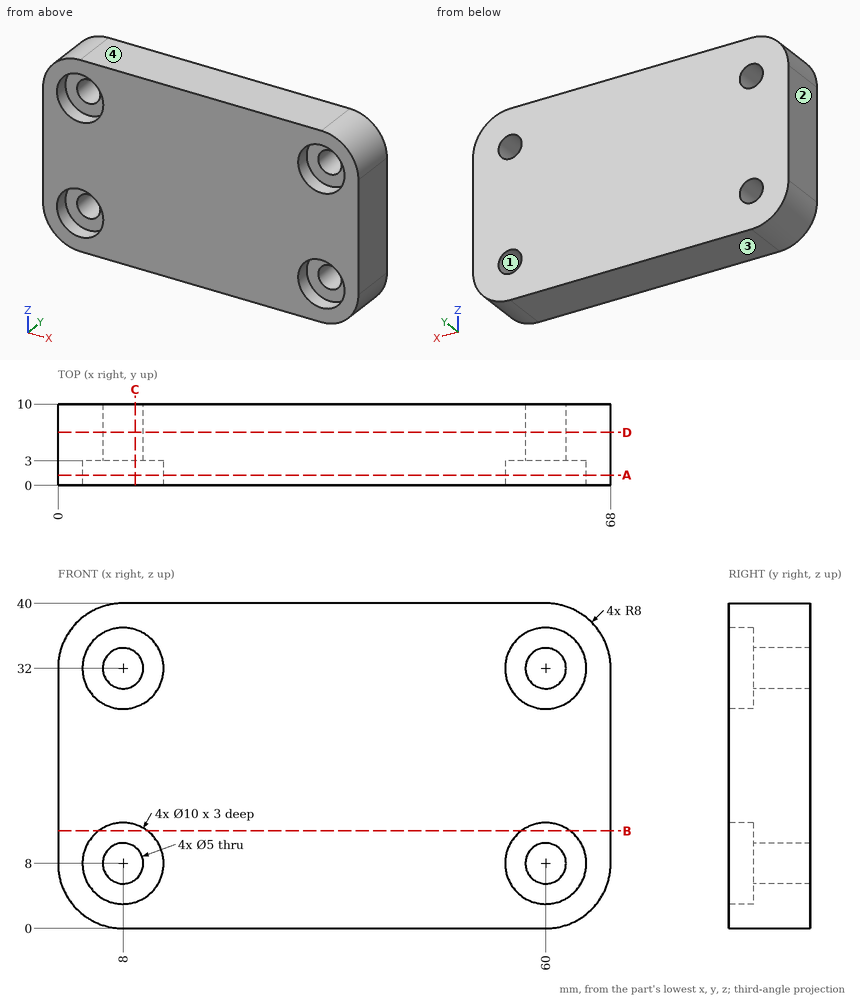
Part print with two shaded views. Sizes in mm from the minimum x, y, z corner. Round coordinates to 2 decimals unless told otherwise and drop trailing zeros. Loops run counter-clockwise (first coordinate to the right, second up) from the corner with the lowest first, then second, coordinate; pieces in that order, holes last. Notation, with made-up numbers: M 66,-24 L 108,-24 A33 cw 108,8 Z; hole C -32,6.5 d4. An arc over 180 degrees is marked long. Return JSON: item names as keys, results as strings. Group by question number.
(1) Wall check: probe 1 along Z at (x, y) = (60, 5.25); probe 2 along Z at (x, y) = (60, 1); probe 3 along X at (y, z) = (2, 8.5). Give the ranges that are in metal, low to high. Write a range as [from, to].
(2) Saw through at C-C, the plane x = 9.5. List the corners of the cut face in (y, z), and give its area (3 significant figures).
(3) Mould opens along Z. For the marked faces 1, 2, 3 and 4 say: +Z half, -Z half, draft (parallel to the pull), parting line (faces both ways), or undercut.
(4) Saw through at D-D, the plane y = 6.5. List the corners of the cut face in (x, z).
(5) Drop a flat-ended pin along its axis: P1, Ø3, axis at x = 7, z = 6, coming from the -Y side. Give the stop position or say it passes through.
(6) Saw through at B-B, the plane z = 12. List the corners of the cut face in (x, y).
(7) Saw through at A-A, the plane y = 1.25. List the corners of the cut face in (x, z), and give its area (3 significant figures).
Answer list:
{
 "1": {"probe 1": "[0, 5.5], [10.5, 29.5], [34.5, 40]", "probe 2": "[0, 3], [13, 27], [37, 40]", "probe 3": "[0, 3.03], [12.97, 55.03], [64.97, 68]"},
 "2": {"outline": "M 0,0 L 10,0 L 10,6 L 3,6 L 3,3.23 L 0,3.23 Z; M 0,12.77 L 3,12.77 L 3,10 L 10,10 L 10,30 L 3,30 L 3,27.23 L 0,27.23 Z; M 0,36.77 L 3,36.77 L 3,34 L 10,34 L 10,40 L 0,40 Z", "area": "287 mm2"},
 "3": {"face 1": "undercut", "face 2": "draft", "face 3": "-Z half", "face 4": "+Z half"},
 "4": {"outline": "M 0,8 A8 ccw 8,0 L 60,0 A8 ccw 68,8 L 68,32 A8 ccw 60,40 L 8,40 A8 ccw 0,32 Z; hole C 8,8 d5; hole C 8,32 d5; hole C 60,8 d5; hole C 60,32 d5"},
 "5": {"P1": "y = 3"},
 "6": {"outline": "M 0,0 L 5,0 L 5,3 L 11,3 L 11,0 L 57,0 L 57,3 L 63,3 L 63,0 L 68,0 L 68,10 L 0,10 Z"},
 "7": {"outline": "M 0,8 A8 ccw 8,0 L 60,0 A8 ccw 68,8 L 68,32 A8 ccw 60,40 L 8,40 A8 ccw 0,32 Z; hole C 8,8 d10; hole C 8,32 d10; hole C 60,8 d10; hole C 60,32 d10", "area": "2,350 mm2"}
}
